```python
from build123d import *

# Parameters (mm, degrees)
HOLE_WIZARD_M51_D = 5.5


with BuildPart() as part:
    # Эскиз1 → Повернуть1 (revolve)
    with BuildSketch(Plane.XY, mode=Mode.PRIVATE) as revolve_1_sk:
        Polygon((13.5, 5), (13.5, 0), (17.5, 0), (17.5, -10), (22.5, -10), (22.5, -5), (32.5, -5), (32.5, 15), (17.5, 15), (17.5, 5), align=None)
    revolve(revolve_1_sk.sketch.rotate(Axis((0, 0, 0), (0, 1, 0)), 90), axis=Axis((0, 0, 0), (0, 1, 0)))

    # Отверстие с зазором M51 (through all)
    with Locations(Plane(origin=(0, 15, 0), x_dir=(-1, 0, 0), z_dir=(0, 1, 0))):
        with Locations((19.445436483, 19.445436483), (19.445436483, -19.445436483), (-19.445436483, -19.445436483), (-19.445436483, 19.445436483)):
            Hole(HOLE_WIZARD_M51_D / 2)


solid = part.part
```
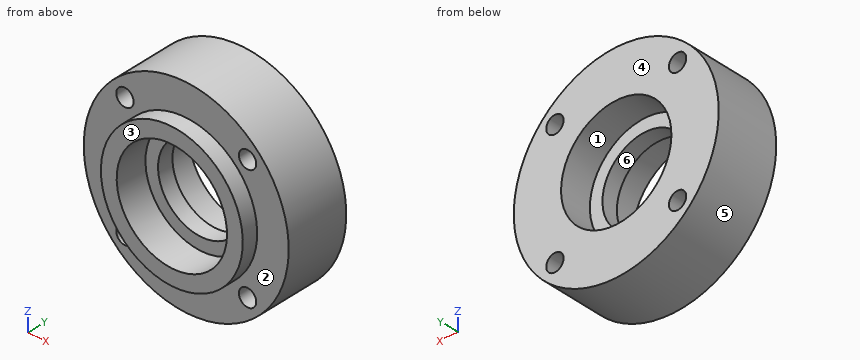
Design review of the part built by this model. Coordinates are the model's own, in mm. Face numbers are marked on the shaded views. A direction names the side the tool comes from. Give positions to 0.01 mm unless a question says otherwise; leave off trailing zeros. Write each loop counter-clockwise with the first axis right and the second up, starting at its lowest first coordinate (ties: lowest second). Pieces come first, ordered by that corner, then holes. Notation, with made-up numbers: (-34.75, 68.5) - (8.25, 68.5) arc R5 ccw to (8.25, 74.5) - close; hole circle Ø1 at (27.25, 2.25). An arc over 180 degrees is marked (long way). Return JSON: item names as keys, results as strings. Group by question number.
(1) We need section B-B, the plane z = 0. Give the boundary of the cut face in (x, y), then the cut area to 3 significant figures.
(2) Mouldability with a two-part tool opening along X and no side actions: class the marked faces 4, 5 and 6 as +X half, -X half, draft (parallel to the pull), parting line (faces both ways), or undercut.
(3) To check wall thickness, follow probe 1 along X at (y, z) = (12.75, 0); probe 2 along X at (y, z) = (-5.25, 0); probe 3 along Y at (x, z) = (29, 10). State the ranges of each line that lie inside material, in increasing order.
(4) We need section C-C, the plane y = -8. Give the boundary of the cut face in (x, z).
(5) Insertion check: pin 1 (3.5 mm diameter, centred on x = 19.45, z = -19.45, fed in from +Y); pin 2 (4 mm diameter, centred on y = -2.5, z = -25, fed in from -X); pin 3 (12 mm diameter, centred on x = -1, y = -0.5, fed in from +Z); pin 4 (6 mm diameter, centred on y = -6.5, z = -10.5, fed in from +X). Each pin has a flat end and moves straight along its axis. Give the tip position at first contact, or say it passes through.
(6) Machinability: for the marked faces 1, 2 and 3, which of the approach directions +Z, -Z, +X, -X, +Y, -Y give a long, thin tool a straight path to every point of the face, cutting with its end or side? Answer none if there is none.
(7) We need section D-D, the plane z = 21. Give the boundary of the cut face in (x, y).
(8) We need section A-A, the plane x = 0. Give the boundary of the cut face in (y, z), then the cut area to 3 significant figures.
Reported:
{
 "1": {"outline": "(-32.5, -5) - (-22.5, -5) - (-22.5, -10) - (-17.5, -10) - (-17.5, 0) - (-13.5, 0) - (-13.5, 5) - (-17.5, 5) - (-17.5, 15) - (-32.5, 15) - close; (13.5, 0) - (17.5, 0) - (17.5, -10) - (22.5, -10) - (22.5, -5) - (32.5, -5) - (32.5, 15) - (17.5, 15) - (17.5, 5) - (13.5, 5) - close", "area": "690 mm2"},
 "2": {"face 4": "draft", "face 5": "parting line", "face 6": "undercut"},
 "3": {"probe 1": "x = -32.5 to -17.5, 17.5 to 32.5", "probe 2": "x = -22.5 to -17.5, 17.5 to 22.5", "probe 3": "y = -5 to 15"},
 "4": {"outline": "circle Ø45 at (0, 0); hole circle Ø35 at (0, 0)"},
 "5": {"pin 1": "passes through", "pin 2": "stops at x = -22.96", "pin 3": "stops at z = 32.5", "pin 4": "stops at x = 31.52"},
 "6": {"face 1": "+Y", "face 2": "-Y", "face 3": "+Z, -Z, +X, -X, -Y"},
 "7": {"outline": "(-24.8, -5) - (-21.71, -5) - (-21.71, 15) - (-24.8, 15) - close; (-17.18, -5) - (-8.08, -5) - (-8.08, -10) - (8.08, -10) - (8.08, -5) - (17.18, -5) - (17.18, 15) - (-17.18, 15) - close; (21.71, -5) - (24.8, -5) - (24.8, 15) - (21.71, 15) - close"},
 "8": {"outline": "(-10, -22.5) - (-5, -22.5) - (-5, -32.5) - (15, -32.5) - (15, -17.5) - (5, -17.5) - (5, -13.5) - (0, -13.5) - (0, -17.5) - (-10, -17.5) - close; (-10, 17.5) - (0, 17.5) - (0, 13.5) - (5, 13.5) - (5, 17.5) - (15, 17.5) - (15, 32.5) - (-5, 32.5) - (-5, 22.5) - (-10, 22.5) - close", "area": "690 mm2"}
}
